Answer from the drawing. Dimensions are ordinates in mm from the lowest x, y and z of the part. Give positions to 0.01 mm unless a question says otherwise; leave off trailing zeros. One line per question, with ' | ' between items. Start each with the question number.
1. Find the intervals of material crossed by line 1 (X direction, y = 7.5, z = 37.5); line 2 (X direction, y = 6.75, z = 46); line 3 (X direction, y = 1.75, z = 24.5) (1 decimal), in increasing order.
2. Section B-B (x = 146) is taken. Give the number of separate pieces and of enclosed holes in the cut face, plus the area to 3 significant figures.
3. This flat-tipped pin is pushed along its axis until it touches: pin 1 (3 mm diameter, centred on x = 121, z = 126, fed in from +Y). Where does it stop, or does it pass through?
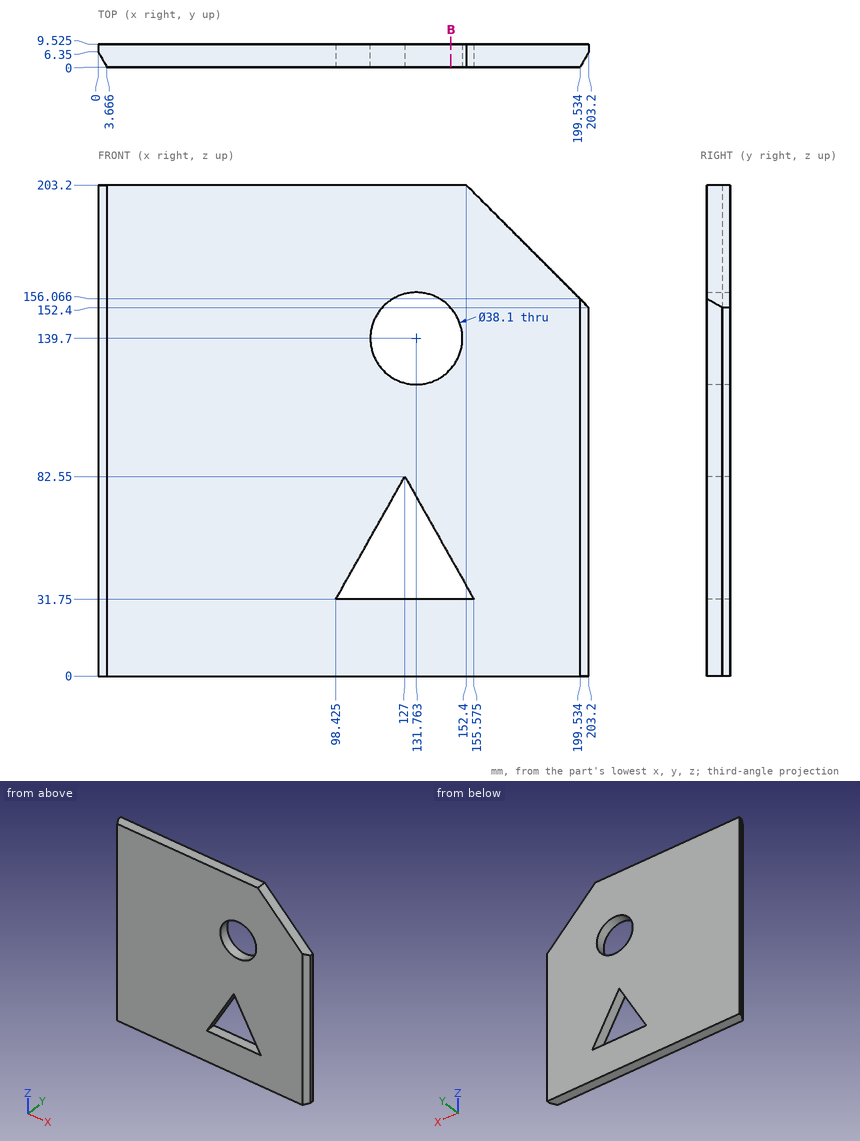
Conclusion:
1) line 1: 0 to 101.66, 152.34 to 203.2 | line 2: 0 to 106.44, 147.56 to 203.2 | line 3: 2.7 to 200.5
2) separate pieces: 3 | enclosed holes: 0 | area: 1,530 mm²
3) pin 1: through
